Design review of the part built by this model. Coordinates are the model's own, in mm. Face numbers are marked on the shaded views. A direction names the side the tool comes from. Coordinates: 2 decimals unless noted, no trailing zeros. Write each loop counter-clockwise with the first axis right and the second up, starting at its lowest first coordinate (ties: lowest second). Pieces come first, ordered by that corner, then holes. Notation, with made-up numbers: (-15, 24) -> (-10, 24) arc R34 ccw to (-10, 61) -> close; hole circle Ø8 at (35, 33.25). An arc over 180 degrees is marked (long way). Answer in a Markdown table with one row per item. Add a question column.
Item 1: Take a section at B-B, the plane y = -7. Write out the cut boundary in (x, z).
Item 2: Clearance check with flat-ended pins moving along their axes: P1, Ø3, axis at y = 6, z = -7.5, coming from the -X side; P2, Ø2.5, axis at x = -13, y = 6, coming from the +Z side; P3, Ø6.5, axis at x = -12, y = -1.5, coming from the -Z side; P4, Ø2.5, axis at x = 14.5, y = -6, coming from the -Z side. State where each tip first meets the part, or that it passes through.
Item 3: Draft analysis for pull direction X (two halves, no side actions). For the marked faces 1, 2, 3 and 4, state which applies: released by +X, released by -X, zero draft, split by the parting line, or undercut.
Item 4: Take a section at D-D, the plane y = 6.5. Write out the cut boundary in (x, z), and give its area (3 significant figures).
Item 5: Take a section at A-A, the plane y = -1.5. Write out the cut boundary in (x, z).
Item 6: For the marked faces 5, 6 and 7, list the 3-axis set-ups (+Z, -Z, +X, -X, +Y, -Y) from which the entire face can be reached by the end or side of a thin tool; tool diameter is ignored.
Item 7: To check wall thickness, follow line 1 (Y direction, x = -13, z = -3.25); line 2 (X direction, y = -6, z = -3.25); line 3 (X direction, y = 6, z = -3.55). State the ranges of each line that lie inside material, in increasing order.
Item 8: Take a section at C-C, the plane x = 0. Write out the cut boundary in (y, z).
from build123d import *

# Parameters (mm, degrees)
F1_DEPTH = 13
F3_DEPTH = 10.501


with BuildPart() as f1:
    # F0 (on Front) → F1 (new body, symmetric)
    with BuildSketch(Plane.XZ):
        with BuildLine():
            ThreePointArc((7.483315, -0.5), (0, -7.5), (-7.483315, -0.5))
            Line((-7.483315, -0.5), (-10.488088, -0.5))
            Line((-10.488088, -0.5), (-17.5, -0.5))
            Line((-17.5, -0.5), (-17.5, -4.5))
            Line((-17.5, -4.5), (-9.486833, -4.5))
            ThreePointArc((-9.486833, -4.5), (0, -10.5), (9.486833, -4.5))
            Line((9.486833, -4.5), (17.5, -4.5))
            Line((17.5, -4.5), (17.5, -0.5))
            Line((17.5, -0.5), (10.488088, -0.5))
            Line((10.488088, -0.5), (7.483315, -0.5))
        make_face()
    extrude(amount=F1_DEPTH, both=True)

    # F2 (on Top) → F3 (cut, through all)
    with BuildSketch(Plane.XY):
        with BuildLine():
            ThreePointArc((14.5, 6), (11.93934, 7.06066), (13, 4.5))
            ThreePointArc((13, 4.5), (14.06066, 4.93934), (14.5, 6))
        make_face()
        with BuildLine():
            ThreePointArc((14.5, -6), (14.06066, -4.93934), (13, -4.5))
            ThreePointArc((13, -4.5), (11.93934, -7.06066), (14.5, -6))
        make_face()
        with BuildLine():
            ThreePointArc((-11.5, 6), (-14.06066, 7.06066), (-13, 4.5))
            ThreePointArc((-13, 4.5), (-11.93934, 4.93934), (-11.5, 6))
        make_face()
        with BuildLine():
            ThreePointArc((-11.5, -6), (-11.93934, -4.93934), (-13, -4.5))
            ThreePointArc((-13, -4.5), (-14.06066, -7.06066), (-11.5, -6))
        make_face()
    extrude(amount=-F3_DEPTH, mode=Mode.SUBTRACT)


solid = f1.part
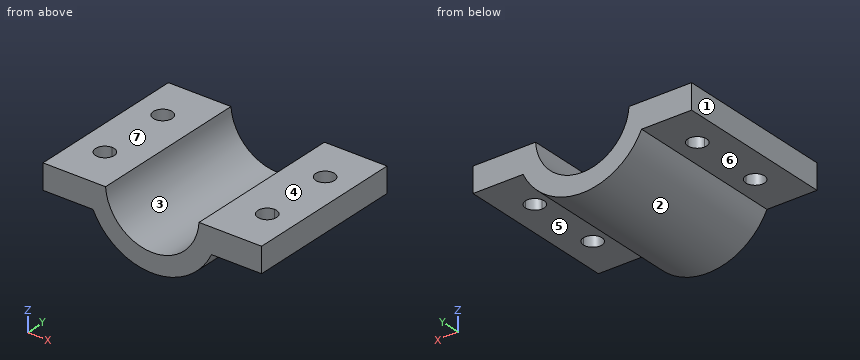
Answers:
| question | item | result |
|---|---|---|
| 1 | outline | (-17.5, -4.5) -> (-14.12, -4.5) -> (-14.12, -0.5) -> (-17.5, -0.5) -> close; (-11.88, -4.5) -> (-9.49, -4.5) arc R10.5 ccw to (9.49, -4.5) -> (11.88, -4.5) -> (11.88, -0.5) -> (7.48, -0.5) arc R7.5 cw to (-7.48, -0.5) -> (-11.88, -0.5) -> close; (14.12, -4.5) -> (17.5, -4.5) -> (17.5, -0.5) -> (14.12, -0.5) -> close |
| 2 | P1 | stops at x = -8.62 |
| 2 | P2 | passes through |
| 2 | P3 | stops at z = -5.8 |
| 2 | P4 | stops at z = -4.5 |
| 3 | face 1 | released by -X |
| 3 | face 2 | split by the parting line |
| 3 | face 3 | undercut |
| 3 | face 4 | zero draft |
| 4 | outline | (-17.5, -4.5) -> (-14.41, -4.5) -> (-14.41, -0.5) -> (-17.5, -0.5) -> close; (-11.59, -4.5) -> (-9.49, -4.5) arc R10.5 ccw to (9.49, -4.5) -> (11.59, -4.5) -> (11.59, -0.5) -> (7.48, -0.5) arc R7.5 cw to (-7.48, -0.5) -> (-11.59, -0.5) -> close; (14.41, -4.5) -> (17.5, -4.5) -> (17.5, -0.5) -> (14.41, -0.5) -> close |
| 4 | area | 118 mm^2 |
| 5 | outline | (-17.5, -4.5) -> (-9.49, -4.5) arc R10.5 ccw to (9.49, -4.5) -> (17.5, -4.5) -> (17.5, -0.5) -> (7.48, -0.5) arc R7.5 cw to (-7.48, -0.5) -> (-17.5, -0.5) -> close |
| 6 | face 5 | -Z, +X, +Y, -Y |
| 6 | face 6 | -Z, -X, +Y, -Y |
| 6 | face 7 | +Z, +X, -X, +Y, -Y |
| 7 | line 1 | y = -13 to -7.5, -4.5 to 4.5, 7.5 to 13 |
| 7 | line 2 | x = -17.5 to -14.5, -11.5 to -6.76, 6.76 to 11.5, 14.5 to 17.5 |
| 7 | line 3 | x = -17.5 to -14.5, -11.5 to -6.61, 6.61 to 11.5, 14.5 to 17.5 |
| 8 | outline | (-13, -10.5) -> (13, -10.5) -> (13, -7.5) -> (-13, -7.5) -> close |
